The listing builds one solid part. Answer for the finished solid, in the listing's coordinates (mm). Round coordinates to 2 decimals unless told otherwise and drop trailing zeros. Write each loop counter-clockwise with the first axis right and the second up, starting at its lowest first coordinate (ties: lowest second). Pieces come first, ordered by that corner, then holes.
Item 1: Each of these flat-tipped pins is pushed along its axis until it touches: pin 1 (4 mm diameter, centred on y = -184.5, z = -2.5, fed in from +X); pin 2 (4 mm diameter, centred on y = 15, z = 0, fed in from -X); pin 3 (3 mm diameter, centred on y = 0.5, z = -1.5, fed in from +X); pin 4 (1.6 mm diameter, centred on y = 20.5, z = 0, fed in from +X). Where does it stop, or does it pass through?
Item 2: Find section A-A on y = 35. Give the vertices of the cut face in (x, z), then the cut area to 3 significant figures.
Item 3: Find the intervals of material crossed by probe 1 along Y at (x, z) = (0.8, 0); probe 2 along Y at (x, z) = (0.7, 0); probe 3 along Y at (x, z) = (17, -3), in increasing order.
Item 4: Find section C-C on x = 15. Give the vertices of the cut face in (y, z), then the cut area to 3 significant figures.
Item 5: Find section B-B on z = 0. Give the vertices of the cut face in (x, y).
```python
from build123d import *

# Parameters (mm, degrees)
SKETCH3_R             = 4
CHAMFER1_SIZE         = 2
CHAMFER1_SIZE2        = 57.272506566
SKETCH4_OUTSIDE_W     = 109.39
SKETCH4_OUTSIDE_H     = 70.198
SKETCH4_OUTSIDE_W_2   = 6
SKETCH4_OUTSIDE_H_2   = 35.530215116
EXTRUDE1_DEPTH        = 30
M6_TAPPED_HOLE1_D     = 5
M6_TAPPED_HOLE1_DEPTH = 9
M6_TAPPED_HOLE1_TIP   = 1.502151548


with BuildPart() as part:
    # Sweep1: sweep along a path in Sketch1
    with BuildLine(Plane.XY) as sweep1_path:
        Line((0, 40), (0, 10))
        ThreePointArc((0, 10), (2.928932188, 2.928932188), (10, 0))
        Line((10, 0), (29.191555041, 0))
        ThreePointArc((29.191555041, 0), (36.531808546, -3.208779308), (39.161411338, -10.775864303))
        Line((39.161411338, -10.775864303), (20, -257))
    # Sketch3 → Sweep1 (sweep)
    with BuildSketch(Plane(origin=(0, 40, 0), x_dir=(1, 0, 0), z_dir=(0, 1, 0))):
        Circle(SKETCH3_R)
    sweep(path=sweep1_path.line)

    # Chamfer1
    chamfer1_edges = [part.edges().sort_by_distance(p)[0] for p in [
        (16.012057481, -256.689654279, 0),
    ]]
    chamfer1_side = [part.faces().sort_by_distance(p)[0] for p in [
        (20, -257, 0),
    ]]
    chamfer(chamfer1_edges, length=CHAMFER1_SIZE, length2=CHAMFER1_SIZE2, reference=chamfer1_side[0])

    # Sketch4 outside → Extrude1 (cut)
    with BuildSketch(Plane(origin=(0, 40, 0), x_dir=(1, 0, 0), z_dir=(0, 1, 0))):
        with Locations((19.596, 0)):
            Rectangle(SKETCH4_OUTSIDE_W, SKETCH4_OUTSIDE_H)
        Rectangle(SKETCH4_OUTSIDE_W_2, SKETCH4_OUTSIDE_H_2, mode=Mode.SUBTRACT)
    extrude(amount=-EXTRUDE1_DEPTH, mode=Mode.SUBTRACT)

    # M6 Tapped Hole1
    with Locations(Plane(origin=(3, 0, 0), x_dir=(0, 0, -1), z_dir=(1, 0, 0))):
        with Locations((0, 35), (0, 15)):
            Hole(M6_TAPPED_HOLE1_D / 2, depth=M6_TAPPED_HOLE1_DEPTH)
            with Locations((0, 0, -(M6_TAPPED_HOLE1_DEPTH + M6_TAPPED_HOLE1_TIP / 2))):  # 118° drill point
                Cone(0, M6_TAPPED_HOLE1_D / 2, M6_TAPPED_HOLE1_TIP, mode=Mode.SUBTRACT)


solid = part.part
```
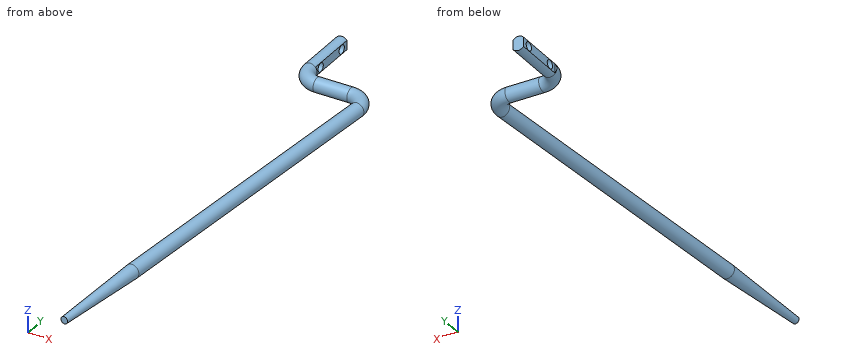
Check values:
1. pin 1: stops at x = 29.66
1. pin 2: passes through
1. pin 3: stops at x = 39.68
1. pin 4: stops at x = 3
2. outline: (-3, -2.65) arc R4 ccw to (3, -2.65) - (3, -2.5) - (-3, -2.5) - close; (-3, 2.5) - (3, 2.5) - (3, 2.65) arc R4 ccw to (-3, 2.65) - close
2. area: 13.0 mm2
3. probe 1: y = -0.55 to 12.5, 17.5 to 32.5, 37.5 to 40
3. probe 2: y = -0.46 to 12.5, 17.5 to 32.5, 37.5 to 40
3. probe 3: y = -2.65 to 2.65
4. outline: circle Ø8 at (0, 0)
4. area: 50.3 mm2
5. outline: (-4, 10) arc R14 ccw to (10, -4) - (29.19, -4) arc R6 cw to (35.17, -10.47) - (20.46, -199.59) - (18.01, -256.84) - (21.99, -257.16) - (28.43, -200.21) - (43.15, -11.09) arc R14 ccw to (29.19, 4) - (10, 4) arc R6 cw to (4, 10) - (3, 10) - (3, 12.5) - (-3, 12.5) - (-3, 10) - close; (-3, 17.5) - (3, 17.5) - (3, 32.5) - (-3, 32.5) - close; (-3, 37.5) - (3, 37.5) - (3, 40) - (-3, 40) - close
